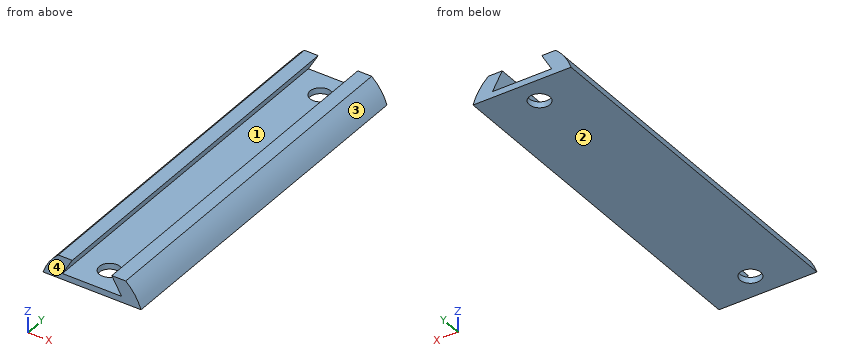
from build123d import *

# Parameters (mm, degrees)
F1_DEPTH = 70
F2_R     = 2
F3_DEPTH = 1.151


with BuildPart() as f1:
    # F0 (on Front) → F1 (new body)
    with BuildSketch(Plane.XZ):
        with BuildLine():
            Line((-9.5, 3.122499), (9.5, 3.122499))
            ThreePointArc((9.5, 3.122499), (8.318707, 5.549695), (6.531252, 7.572499))
            Line((6.531252, 7.572499), (3.831252, 7.572499))
            Line((3.831252, 7.572499), (5.736508, 4.272499))
            Line((5.736508, 4.272499), (0, 4.272499))
            Line((0, 4.272499), (-5.736508, 4.272499))
            Line((-5.736508, 4.272499), (-3.831252, 7.572499))
            Line((-3.831252, 7.572499), (-6.531252, 7.572499))
            ThreePointArc((-6.531252, 7.572499), (-8.318707, 5.549695), (-9.5, 3.122499))
        make_face()
    extrude(amount=-F1_DEPTH)

    # F2 (on face) → F3 (cut, through all)
    with BuildSketch(Plane.XY.offset(4.272499)):
        with Locations((0, 5)):
            Circle(F2_R)
        with Locations((0, 65)):
            Circle(F2_R)
    extrude(amount=-F3_DEPTH, mode=Mode.SUBTRACT)


solid = f1.part
For this review, take the finished solid that the model builds, in its own axes (mm). Face numbers are marked on the shaded views. Give positions to 0.01 mm unless a question says otherwise; leave off trailing zeros. Order: outer loops, then holes, each group sorted by start corner. A loop starts at its lowest first (then second) coordinate and runs counter-clockwise, first axis right, second up. Notation, with made-up numbers: M 46,17.25 L 56,17.25 A32 ccw 56,54.25 Z; hole C 59,43.5 d4. An arc over 180 degrees is marked long. Answer in a Markdown table with one row per item. Add a question column.
(1) Consider section B-B on y = 65. State the section outline as (x, z) points.
(2) Consider section C-C on z = 6.6. State the section outline as (x, y) points.
(3) Consider section A-A on x = 0. State the section outline as (y, z) points, and give its area (3 significant figures).
(4) For pin 1 (6 mm diameter, centred on x = -2, y = 40, fed in from +Z); pin 2 (1 mm diameter, centred on y = 31.5, z = 4.5, fed in from +X); pin 3 (4.5 mm diameter, centred on x = 0, y = 65, fed in from +Z), all flat-tipped, find the tip position at first contact; note any pin that passes through.
(5) Wall thickness on probe 1 along Y at (x, z) = (0, 3.75); probe 2 along Z at (x, y) = (-3, 33); probe 3 along X at (y, z) = (52.5, 7.4): over which ranges is each line inside the solid? List them lowest first. Write a range as [from, to].
(6) Consider section D-D on y = 42. State the section outline as (x, z) points, and give its area (3 significant figures).
(7) Mouldability with a two-part tool opening along Z and no side actions: class the marked faces 1, 2, 3 and 4 as +Z half, -Z half, draft (parallel to the pull), parting line (faces both ways), or undercut.
Evaluation:
| question | item | result |
|---|---|---|
| 1 | outline | M -9.5,3.12 L -2,3.12 L -2,4.27 L -5.74,4.27 L -3.83,7.57 L -6.53,7.57 A10 ccw Z; M 2,3.12 L 9.5,3.12 A10 ccw 6.53,7.57 L 3.83,7.57 L 5.74,4.27 L 2,4.27 Z |
| 2 | outline | M -7.51,0 L -4.39,0 L -4.39,70 L -7.51,70 Z; M 4.39,0 L 7.51,0 L 7.51,70 L 4.39,70 Z |
| 3 | outline | M 0,3.12 L 3,3.12 L 3,4.27 L 0,4.27 Z; M 7,3.12 L 63,3.12 L 63,4.27 L 7,4.27 Z; M 67,3.12 L 70,3.12 L 70,4.27 L 67,4.27 Z |
| 3 | area | 71.3 mm^2 |
| 4 | pin 1 | stops at z = 7.57 |
| 4 | pin 2 | stops at x = 9.17 |
| 4 | pin 3 | stops at z = 4.27 |
| 5 | probe 1 | y = [0, 3], [7, 63], [67, 70] |
| 5 | probe 2 | z = [3.12, 4.27] |
| 5 | probe 3 | x = [-6.73, -3.93], [3.93, 6.73] |
| 6 | outline | M -9.5,3.12 L 9.5,3.12 A10 ccw 6.53,7.57 L 3.83,7.57 L 5.74,4.27 L -5.74,4.27 L -3.83,7.57 L -6.53,7.57 A10 ccw Z |
| 6 | area | 42.4 mm^2 |
| 7 | face 1 | undercut |
| 7 | face 2 | -Z half |
| 7 | face 3 | +Z half |
| 7 | face 4 | draft |
